```python
from build123d import *

# Parameters (mm, degrees)
SKETCH2_W           = 1250
SKETCH2_H           = 1250
BOSS_EXTRUDE1_DEPTH = 50
SKETCH3_R           = 500
BOSS_EXTRUDE2_DEPTH = 500
SKETCH4_R           = 25
CUT_EXTRUDE1_DEPTH  = 1016.504800579
SKETCH5_R           = 125
BOSS_EXTRUDE3_DEPTH = 100


with BuildPart() as part:
    # Sketch2 → Boss-Extrude1 (new body)
    with BuildSketch(Plane.XY):
        Rectangle(SKETCH2_W, SKETCH2_H)
    extrude(amount=BOSS_EXTRUDE1_DEPTH)

    # Sketch3 → Boss-Extrude2 (add)
    with BuildSketch(Plane.XY.offset(50)):
        Circle(SKETCH3_R)
    extrude(amount=BOSS_EXTRUDE2_DEPTH)

    # Sketch4 → Cut-Extrude1 (cut, through all)
    with BuildSketch(Plane.XY.offset(50)):
        with Locations((-525, 525)):
            Circle(SKETCH4_R)
        with Locations((-525, -525)):
            Circle(SKETCH4_R)
        with Locations((525, -525)):
            Circle(SKETCH4_R)
        with Locations((525, 525)):
            Circle(SKETCH4_R)
    extrude(amount=-CUT_EXTRUDE1_DEPTH, mode=Mode.SUBTRACT)

    # Sketch5 → Boss-Extrude3 (add)
    with BuildSketch(Plane.XY.offset(550)):
        Circle(SKETCH5_R)
    extrude(amount=BOSS_EXTRUDE3_DEPTH)


solid = part.part
```
Could you check a few things on this model? Use its own coordinates, in mm. A direction names the side the tool comes from. Round coordinates to 2 decimals unless told otherwise and drop trailing zeros. Write each loop counter-clockwise with the first axis right and the second up, starting at its lowest first coordinate (ties: lowest second). Pieces come first, ordered by that corner, then holes. Notation, with made-up numbers: M 19.5,-28.75 L 25.5,-28.75 A20 cw 25.5,-13.75 Z; hole C 42,60.25 d1. An arc over 180 degrees is marked long. Write each question's results on one line, items separated by ' | '. Start each with the question number.
1. I'm going to push flat-ended pins straight in: pin 1 Ø10 at (y, z) = (-444.5, 333) entering from -X; pin 2 Ø12 at (x, z) = (248.5, 292.5) entering from +Y; pin 3 Ø4 at (y, z) = (378.5, 122.5) entering from +X. Where does each tip first touch, or does it pass through?
2. Imagine slicing it at C-C on y = 0. List the corners of the cut face in (x, z) for me.
3. Imagine slicing it at A-A on y = 525. List the corners of the cut face in (x, z) for me.
4. On a 3-axis mill with a long thin cutter (end or side, diameter ignored), from which of +Z, -Z, +X, -X, +Y, -Y can I reach the whole of each face in a straight line? I mean faces 1 (the face through (-2, 2, 650)), 2 (the face through (104, -104, 550)). Say none if no direction works.
5. Thinking about a two-plate mould opening in X: for faces 3 (the face through (625, -9, 25)), 4 (the face through (-124.88, 5.5, 599.3)), 5 (the face through (548.846, 532.509, 25.35)), which applies, +X half, -X half, draft (parallel to the pull), parting line (faces both ways), or undercut?
6. Imagine slicing it at D-D on z = 573.5. List the corners of the cut face in (x, y) for me.
7. I need wall thicknesses on L1, parallel to Y at x = -525, z = 24.5; L2, parallel to Z at x = -22, y = -260; L3, parallel to Z at x = 534.5, y = -279.5. Which ranges of each line are inside material? Lowest first, please. Write a range as from..to.
Result sheet:
1) pin 1: stops at x = -238.41 | pin 2: stops at y = 437.26 | pin 3: stops at x = 329.01
2) outline: M -625,0 L 625,0 L 625,50 L 500,50 L 500,550 L 125,550 L 125,650 L -125,650 L -125,550 L -500,550 L -500,50 L -625,50 Z
3) outline: M -625,0 L -550,0 L -550,50 L -625,50 Z; M -500,0 L 500,0 L 500,50 L -500,50 Z; M 550,0 L 625,0 L 625,50 L 550,50 Z
4) face 1: +Z, +X, -X, +Y, -Y | face 2: +Z
5) face 3: +X half | face 4: parting line | face 5: undercut
6) outline: C 0,0 d250
7) L1: y = -625..-550, -500..500, 550..625 | L2: z = 0..550 | L3: z = 0..50
